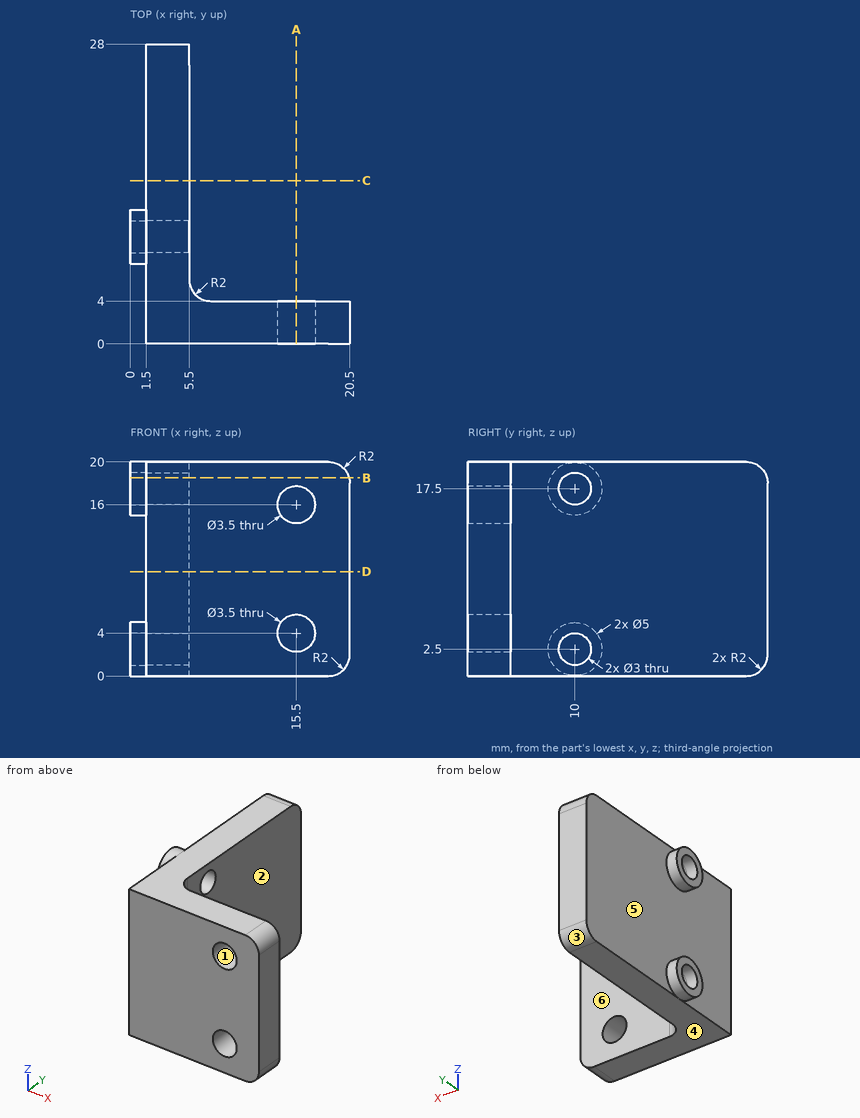
Job drawing, mm, ordinate dimensions from the low corner. One solid piece. A direction names the side the tool comes from. Round coordinates to 2 decimals unless told otherwise and drop trailing zeros. Write each loop counter-clockwise with the first axis right and the second up, starting at its lowest first coordinate (ties: lowest second). Pieces come first, ordered by that corner, then holes. Notation, with made-up numbers: (77.25, -20) -> (85.25, -20) arc R13 cw to (85.25, -12) -> close; hole circle Ø1 at (9, 0.5). An arc over 180 degrees is marked (long way). Answer as CSV lines item,"result".
1. Slice it at A-A, the plane x = 15.5. List the corners of the cut face in (y, z), plus the area to 3 significant figures.
Resolved:
outline,"(0, 0) -> (4, 0) -> (4, 2.25) -> (0, 2.25) -> close; (0, 5.75) -> (4, 5.75) -> (4, 14.25) -> (0, 14.25) -> close; (0, 17.75) -> (4, 17.75) -> (4, 20) -> (0, 20) -> close"
area,"52.0 mm²"
2. Slice it at C-C, the plane y = 15.25. List the corners of the cut face in (x, z).
Resolved:
outline,"(1.5, 0) -> (5.5, 0) -> (5.5, 20) -> (1.5, 20) -> close"
3. Tool access for the marked faces 4, 5 and 6: list every direction of +Z, -Z, +X, -X, +Y, -Y with a clear straight run to the whole face (end or side of a thin tool).
Resolved:
face 4,"-Z, +X, -X, +Y, -Y"
face 5,"-X"
face 6,"+Z, -Z, +X, +Y"
4. Slice it at B-B, the plane z = 18.5. List the corners of the cut face in (x, y).
Resolved:
outline,"(0, 7.71) -> (1.5, 7.71) -> (1.5, 0) -> (20.44, 0) -> (20.44, 4) -> (7.5, 4) arc R2 cw to (5.5, 6) -> (5.5, 8.88) -> (0, 8.88) -> close; (0, 11.12) -> (5.5, 11.12) -> (5.5, 27.94) -> (1.5, 27.94) -> (1.5, 12.29) -> (0, 12.29) -> close"
5. Pin check, flat tips, straight feed: pin 1 Ø6 at (y, z) = (8.5, 9) entering from -X; pin 2 Ø3.5 at (y, z) = (10, 17.5) entering from +X; pin 3 Ø3 at (x, z) = (12.5, 12) entering from +Y; pin 4 Ø5 at (x, y) = (15.5, 7) entering from -Z. Stop position of each tip, or through.
Resolved:
pin 1,"x = 1.5"
pin 2,"x = 5.5"
pin 3,"y = 4"
pin 4,"through"
6. Slice it at D-D, the plane z = 9.75. List the corners of the cut face in (x, y).
Resolved:
outline,"(1.5, 0) -> (20.5, 0) -> (20.5, 4) -> (7.5, 4) arc R2 cw to (5.5, 6) -> (5.5, 28) -> (1.5, 28) -> close"
7. Mould opens along Z. For the marked faces 1, 2 and 3 say: +Z half, -Z half, draft (parallel to the pull), parting line (faces both ways), or undercut.
Resolved:
face 1,"undercut"
face 2,"draft"
face 3,"-Z half"
8. Drill centre lines: line 1 (X direction, y = 14.5, z = 9.75); line 2 (Y direction, x = 11, z = 11); line 3 (Y direction, x = 1.1, z = 17.5). Where is each one in solid material? Low to high.
Resolved:
line 1,"1.5 to 5.5"
line 2,"0 to 4"
line 3,"7.5 to 8.5, 11.5 to 12.5"
